from build123d import *

# Parameters (mm, degrees)
SKETCH1_R           = 7
BOSS_EXTRUDE1_DEPTH = 45


with BuildPart() as part:
    # Sketch1 → Boss-Extrude1 (new body)
    with BuildSketch(Plane.XY):
        with BuildLine():
            Line((0, 0), (-7, 7))
            Line((-7, 7), (-7, 25))
            Line((-7, 25), (0, 32))
            Line((0, 32), (7, 32))
            Line((7, 32), (33.868127266, 27.262424242))
            ThreePointArc((33.868127266, 27.262424242), (44.39557659, 28.402372071), (52.677966102, 35))
            Line((52.677966102, 35), (76.505552309, 35))
            Line((76.505552309, 35), (81.677966102, 30))
            Line((81.677966102, 30), (82, 11))
            Line((82, 11), (53, -19))
            Line((53, -19), (49.457764366, -19))
            ThreePointArc((49.457764366, -19), (45.01879217, -12.115672061), (42.681961966, -4.264705882))
            ThreePointArc((42.681961966, -4.264705882), (41.001559006, -1.213413768), (37.736323225, 0))
            Line((37.736323225, 0), (0, 0))
        make_face()
        with Locations(Location((7, 14, 0), (0, 0, 180))):
            Circle(SKETCH1_R, mode=Mode.SUBTRACT)
    extrude(amount=BOSS_EXTRUDE1_DEPTH)


solid = part.part
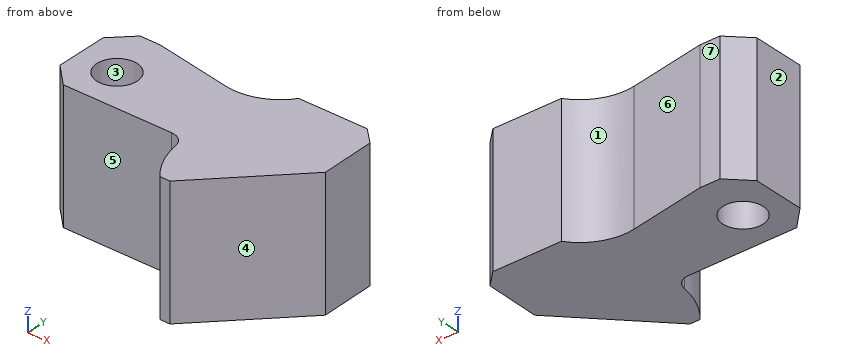
CAD build for the part. Positions are in the model's coordinates, mm. Face numbers are marked on the shaded views. A direction names the side the tool comes from. Coordinates: 2 decimals unless noted, no trailing zeros. Loops run counter-clockwise (first coordinate to the right, second up) from the corner with the lowest first, then second, coordinate; pieces in that order, holes last. Notation, with made-up numbers: (14.5, 84) - (25.5, 84) arc R22 ccw to (25.5, 112) - close; hole circle Ø2 at (-13, -21). An arc over 180 degrees is marked (long way). Write item = value, one per line. Start each with the question number.
Q1. Flat gauge pins, fed straight in: pin 1 Ø4 at (y, z) = (21, 19) entering from +X; pin 2 Ø7.5 at (x, z) = (4, 25) entering from +Y; pin 3 Ø11.5 at (x, z) = (28, 19.5) entering from -Y. Where does each tip first touch, or does it go through?
Q2. Cut at C-C, the plane x = 72. List the corners of the cut face in (y, z), then the cut area to 3 significant figures.
Q3. Cut at A-A, the plane z = 15. List the corners of the cut face in (x, y).
Q4. Pull direction Y, two halves, no side cores. Call the marked faces 1, 2, 3 and 4: pulls with the +Y half, pulls with the -Y half, needs draft (parallel to the pull), parting line crosses it, or undercut.
Q5. Cut at D-D, the plane y = -13.5. List the corners of the cut face in (x, z).
Q6. Which spindle directions (+Z, -Z, +X, -X, +Y, -Y) get a long thin tool onto all of the face, cutting with end or side? Do the marked faces 5, 6 and 7. Say none if no direction does.
Q7. Drill centre lines: L1, parallel to Y at x = 7, z = 31; L2, parallel to X at y = 17, z = 30.5; L3, parallel to X at y = 14, z = 23. Where is each one in solid material? Low to high.
Q8. Cut at B-B, the plane y = 17. List the corners of the cut face in (x, z).
Computed:
q1.pin_1 = 81.86
q1.pin_2 = 32
q1.pin_3 = 0
q2.outline = (0.66, 0) - (35, 0) - (35, 45) - (0.66, 45) - close
q2.area = 1,550 mm²
q3.outline = (-7, 7) - (0, 0) - (37.74, 0) arc R5 cw to (42.68, -4.26) arc R29 ccw to (49.46, -19) - (53, -19) - (82, 11) - (81.68, 30) - (76.51, 35) - (52.68, 35) arc R19 cw to (33.87, 27.26) - (7, 32) - (0, 32) - (-7, 25) - close; hole circle Ø14 at (7, 14)
q4.face_1 = pulls with the +Y half
q4.face_2 = needs draft
q4.face_3 = undercut
q4.face_4 = pulls with the -Y half
q5.outline = (45.7, 0) - (58.32, 0) - (58.32, 45) - (45.7, 45) - close
q6.face_5 = +Z, -Z, -X, -Y
q6.face_6 = +Z, -Z, +Y
q6.face_7 = +Z, -Z, -X, +Y
q7.L1 = 0 to 7, 21 to 32
q7.L2 = -7 to 0.68, 13.32 to 81.9
q7.L3 = -7 to 0, 14 to 81.95
q8.outline = (-7, 0) - (0.68, 0) - (0.68, 45) - (-7, 45) - close; (13.32, 0) - (81.9, 0) - (81.9, 45) - (13.32, 45) - close
